Input: part model. Units: mm. Frame: model coordinates. A direction names the side the tool comes from. Round coordinates to 2 decimals unless told otherwise and drop trailing zeros. Loops run counter-clockwise (first coordinate to the right, second up) from the corner with the lowest first, then second, coordinate; pieces in that order, holes last.
1) Ray query, line 1 along X through (y, z) = (-204.5, -74); line 2 along X through (y, z) = (-48.5, -114); line 3 along Y through (x, z) = (160, -43.5). Return the intervals inside material, ascending.
2) Draft query along X for faces 1 (the face through (572.122, 461, -101)), 2 (the face through (412.122, -157, -57)), 3 (the face through (762.122, 183, -57)), 4 (the face through (493.24, -208.95, -73.95)). Return one class per face: pulls with the +X half, pulls with the -X half, needs draft (parallel to the pull), parting line crosses it, or undercut.
3) Section D-D, the plane z = -117. Return loops of the section in (x, y), and give its area (3 significant figures).
4) Access query for faces 5 (the face through (587.33, 543.25, -69.02)), 6 (the face through (301, 190, -101)), 7 (the face through (587.33, -187.87, -70.98)), 8 (the face through (295, 0, -41)), 9 (the face through (681, 173, -150)). Directions: +Z, -Z, +X, -X, +Y, -Y. A direction counts if a zero-diameter tool reaches every point of the face in a straight line with its end or side. Return the directions, or none.
5) Section B-B, the plane z = -47. Return loops of the section in (x, y), and give its area (3 significant figures).
6) Section A-A, the plane y = 107.5. Return loops of the section in (x, z), and give its area (3 significant figures).
7) First-contact query: pin 1 (6 mm diameter, centred on y = -192.5, z = -34.5, fed in from -X); pin 2 (12 mm diameter, centred on x = 655, y = -203, fed in from -Z); pin 3 (4 mm diameter, centred on x = 228.5, y = 297, fed in from +Z). Flat tips, straight axial feed; report the tip coordinate or a pass-through.
8) Section C-C, the plane x = 356. Return loops of the section in (y, z).
from build123d import *

# Parameters (mm, degrees)
BOSS_EXTRUDE1_DEPTH = 350
SKETCH2_W           = 150
SKETCH2_H           = 350
BOSS_EXTRUDE2_DEPTH = 350
BOSS_EXTRUDE3_DEPTH = 350
BOSS_EXTRUDE4_DEPTH = 350
SKETCH6_W           = 438.570660024
SKETCH6_H           = 30
CUT_EXTRUDE1_DEPTH  = 10
CUT_EXTRUDE2_DEPTH  = 10
SKETCH8_W           = 30
SKETCH8_H           = 438.570660025
CUT_EXTRUDE3_DEPTH  = 10
SKETCH9_W           = 30
SKETCH9_H           = 438.570660025
CUT_EXTRUDE4_DEPTH  = 10


with BuildPart() as part:
    # Sketch1 → Boss-Extrude1 (new body)
    with BuildSketch(Plane(origin=(0, 0, 0), x_dir=(1, 0, 0), z_dir=(0, 1, 0))):
        Polygon((0, 0), (412.121612918, 0), (412.121612918, 150), align=None)
    extrude(amount=BOSS_EXTRUDE1_DEPTH)

    # Sketch2 → Boss-Extrude2 (add)
    with BuildSketch(Plane(origin=(412.121612918, 0, 0), x_dir=(0, 0, -1), z_dir=(1, 0, 0))):
        with Locations((75, 175)):
            Rectangle(SKETCH2_W, SKETCH2_H)
    extrude(amount=BOSS_EXTRUDE2_DEPTH)

    # Sketch4 → Boss-Extrude3 (add)
    with BuildSketch(Plane(origin=(762.121612918, 0, 0), x_dir=(0, 0, -1), z_dir=(1, 0, 0))):
        Polygon((0, 762.121612918), (150, 350), (0, 350), align=None)
    extrude(amount=-BOSS_EXTRUDE3_DEPTH)

    # Sketch5 → Boss-Extrude4 (add)
    with BuildSketch(Plane(origin=(762.121612918, 0, 0), x_dir=(0, 0, -1), z_dir=(1, 0, 0))):
        Polygon((0, 0), (0, -412.121612918), (150, 0), align=None)
    extrude(amount=-BOSS_EXTRUDE4_DEPTH)

    # Sketch6 → Cut-Extrude1 (cut)
    with BuildSketch(Plane(origin=(0, 0, 0), x_dir=(-0.9396926207859104, 0, 0.34202014332566316), z_dir=(-0.34202014332566316, 0, -0.9396926207859104))):
        with Locations((-219.285330012, 175)):
            Rectangle(SKETCH6_W, SKETCH6_H)
    extrude(amount=-CUT_EXTRUDE1_DEPTH, mode=Mode.SUBTRACT)

    # Sketch7 → Cut-Extrude2 (cut)
    with BuildSketch(Plane(origin=(0, 0, -150), x_dir=(-1, 0, 0), z_dir=(0, 0, -1))):
        Polygon((-412.121612918, 190), (-572.121612918, 190), (-572.121612918, 350), (-602.121612918, 350), (-602.121612918, 190), (-602.121612918, 164.900861359), (-602.121612918, 160), (-602.121612918, 0), (-572.121612918, 0), (-572.121612918, 160), (-412.121612918, 160), align=None)
    extrude(amount=-CUT_EXTRUDE2_DEPTH, mode=Mode.SUBTRACT)

    # Sketch8 → Cut-Extrude3 (cut)
    with BuildSketch(Plane(origin=(0, -48.209070726, -132.453333234), x_dir=(-1, 0, 0), z_dir=(0, -0.34202014332566283, -0.9396926207859106))):
        with Locations((-587.121612918, -167.982308514)):
            Rectangle(SKETCH8_W, SKETCH8_H)
    extrude(amount=-CUT_EXTRUDE3_DEPTH, mode=Mode.SUBTRACT)

    # Sketch9 → Cut-Extrude4 (cut)
    with BuildSketch(Plane(origin=(0, 89.151293181, -244.941164929), x_dir=(-1, 0, 0), z_dir=(0, 0.342020143325663, -0.9396926207859105))):
        with Locations((-587.121612918, 496.874725788)):
            Rectangle(SKETCH9_W, SKETCH9_H)
    extrude(amount=-CUT_EXTRUDE4_DEPTH, mode=Mode.SUBTRACT)


solid = part.part
Final values:
1. line 1: x = 412.12 to 572.12, 602.12 to 762.12
1. line 2: x = 412.12 to 762.12
1. line 3: y = 0 to 350
2. face 1: undercut
2. face 2: pulls with the -X half
2. face 3: pulls with the +X half
2. face 4: needs draft
3. outline: (321.45, 0) - (412.12, 0) - (412.12, -90.67) - (572.12, -90.67) - (572.12, -61.43) - (602.12, -61.43) - (602.12, -90.67) - (762.12, -90.67) - (762.12, 440.67) - (602.12, 440.67) - (602.12, 411.43) - (572.12, 411.43) - (572.12, 440.67) - (412.12, 440.67) - (412.12, 350) - (321.45, 350) - (321.45, 190) - (350.69, 190) - (350.69, 160) - (321.45, 160) - close
3. area: 215,000 mm2
4. face 5: -Z, +Y
4. face 6: -Z, -X
4. face 7: -Z, -Y
4. face 8: +Z, -Z, -X, -Y
4. face 9: -Z, +X, -X, +Y, -Y
5. outline: (129.13, 0) - (412.12, 0) - (412.12, -282.99) - (572.12, -282.99) - (572.12, -253.75) - (602.12, -253.75) - (602.12, -282.99) - (762.12, -282.99) - (762.12, 632.99) - (602.12, 632.99) - (602.12, 603.75) - (572.12, 603.75) - (572.12, 632.99) - (412.12, 632.99) - (412.12, 350) - (129.13, 350) - (129.13, 190) - (158.37, 190) - (158.37, 160) - (129.13, 160) - close
5. area: 417,000 mm2
6. outline: (0, 0) - (412.12, -150) - (572.12, -150) - (572.12, -140) - (602.12, -140) - (602.12, -150) - (762.12, -150) - (762.12, 0) - close
6. area: 83,100 mm2
7. pin 1: stops at x = 412.12
7. pin 2: stops at z = -78.3
7. pin 3: stops at z = 0
8. outline: (0, -129.57) - (160, -129.57) - (160, -118.93) - (190, -118.93) - (190, -129.57) - (350, -129.57) - (350, 0) - (0, 0) - close
